Check sheet for the drawn part. Datum: minimum x, y, z corner. Units: mm. Round coordinates to 2 decimals unless told otherwise and drop trailing zeros. Order: outer loops, then holes, each group sorted by start corner. A loop starts at its lowest first (then second) coordinate and runs counter-clockwise, first axis right, second up. Notation, with made-up numbers: M 68,4 L 75,4 A35 cw 75,37 Z; hole C -18.75,-14 d3. An arc over 180 degrees is marked long. Use one line per item in the form item = value. Start each with the question number.
Item 1: Thickness scan on probe 1 along Y at (x, z) = (1.8, 24); probe 2 along Z at (x, y) = (2.5, 6.35) (3 decimals); probe 3 along Y at (x, z) = (0.3, 4.5). Record the ranges inside material, lowest first. Write a range as [from, to].
Item 2: Cross-section at C-C on y = 6.35. Enter the section's corners in (x, z) (3 decimals).
Item 3: Cross-section at B-B on x = 1.3. Enter the section's corners in (y, z) (3 decimals), then the cut area to 3 significant figures.
Item 4: Cross-section at A-A on z = 3.81. Enter the section's corners in (x, y) (3 decimals).
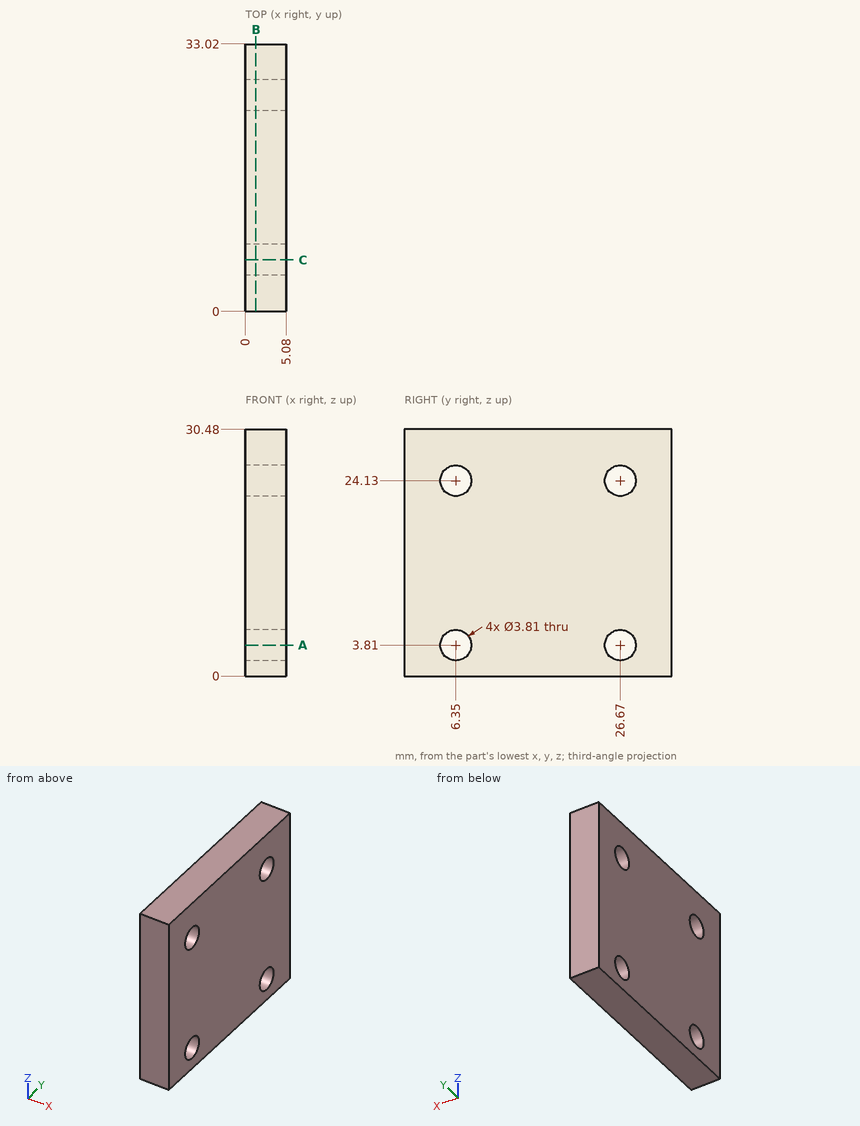
Output values:
q1.probe_1 = [0, 4.45], [8.25, 24.77], [28.57, 33.02]
q1.probe_2 = [0, 1.905], [5.715, 22.225], [26.035, 30.48]
q1.probe_3 = [0, 4.57], [8.13, 24.89], [28.45, 33.02]
q2.outline = M 0,0 L 5.08,0 L 5.08,1.905 L 0,1.905 Z; M 0,5.715 L 5.08,5.715 L 5.08,22.225 L 0,22.225 Z; M 0,26.035 L 5.08,26.035 L 5.08,30.48 L 0,30.48 Z
q3.outline = M 0,0 L 33.02,0 L 33.02,30.48 L 0,30.48 Z; hole C 6.35,3.81 d3.81; hole C 6.35,24.13 d3.81; hole C 26.67,3.81 d3.81; hole C 26.67,24.13 d3.81
q3.area = 961 mm2
q4.outline = M 0,0 L 5.08,0 L 5.08,4.445 L 0,4.445 Z; M 0,8.255 L 5.08,8.255 L 5.08,24.765 L 0,24.765 Z; M 0,28.575 L 5.08,28.575 L 5.08,33.02 L 0,33.02 Z
